Read the model definition and answer for the solid it produces. Units are mm, in the model's axes. Face numbers are marked on the shaded views. A direction names the side the tool comes from. Round coordinates to 2 decimals unless told otherwise and drop trailing zeros. Write each loop counter-clockwise with the first axis right and the second up, starting at its lowest first coordinate (ties: lowest second). Pieces come first, ordered by that corner, then holes.
from build123d import *

# Parameters (mm, degrees)
F0_W     = 75
F0_H     = 25
F0_R     = 1.75
F1_DEPTH = 2
F2_W     = 30
F2_H     = 25
F2_R     = 2.25
F3_DEPTH = 12
F4_DEPTH = 4
F5_R     = 5


with BuildPart() as f1:
    # F0 (on Top) → F1 (new body, symmetric)
    with BuildSketch(Plane.XY):
        Rectangle(F0_W, F0_H)
        with Locations((-30, 0)):
            Circle(F0_R, mode=Mode.SUBTRACT)
        with Locations((-20, 0)):
            Circle(F0_R, mode=Mode.SUBTRACT)
    extrude(amount=F1_DEPTH, both=True)

    # F2 (on face) → F3 (join)
    with BuildSketch(Plane(origin=(0, 0, -2), x_dir=(1, 0, 0), z_dir=(0, 0, -1))):
        with Locations((22.5, 0)):
            Rectangle(F2_W, F2_H)
        with Locations((15, 0)):
            Circle(F2_R, mode=Mode.SUBTRACT)
        with Locations((30, 0)):
            Circle(F2_R, mode=Mode.SUBTRACT)
    extrude(amount=F3_DEPTH)

    # F4 (cut, through all): faces of the model
    f4_faces = [f1.faces().sort_by_distance(p)[0] for p in [
        (15, 0, -2),
        (30, 0, -2),
    ]]
    extrude(f4_faces, amount=-F4_DEPTH, mode=Mode.SUBTRACT)

    # F5
    f5_edges = [f1.edges().sort_by_distance(p)[0] for p in [
        (-37.5, 12.5, 0),
        (-37.5, -12.5, 0),
        (7.5, 0, -2),
        (37.5, -12.5, -6),
        (37.5, 12.5, -6),
    ]]
    fillet(f5_edges, radius=F5_R)


solid = f1.part
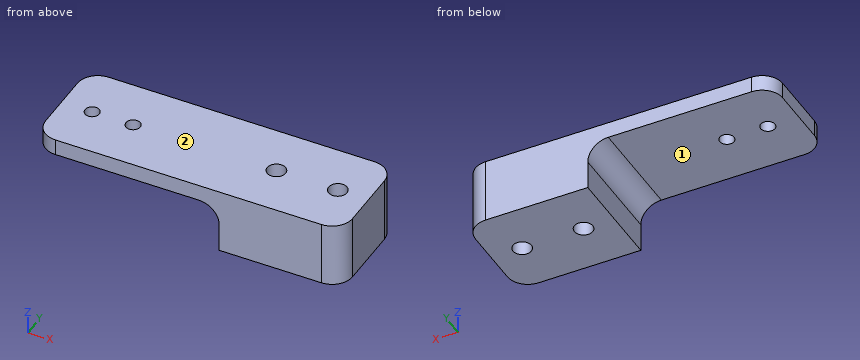
Q1. Section A-A (x = -30) is taken. Determine the outline of the cut face in (y, z).
Verdict:
outline: (-12.5, -2) - (-1.75, -2) - (-1.75, 2) - (-12.5, 2) - close; (1.75, -2) - (12.5, -2) - (12.5, 2) - (1.75, 2) - close
Q2. Section D-D (z = -12.5) is taken. Determine the outline of the cut face in (x, y).
Verdict:
outline: (7.5, -12.5) - (32.5, -12.5) arc R5 ccw to (37.5, -7.5) - (37.5, 7.5) arc R5 ccw to (32.5, 12.5) - (7.5, 12.5) - close; hole circle Ø4.5 at (15, 0); hole circle Ø4.5 at (30, 0)
Q3. Section C-C (z = -0.25) is taken. Determine the outline of the cut face in (x, y), then the cut area to 3 significant figures.
Verdict:
outline: (-37.5, -7.5) arc R5 ccw to (-32.5, -12.5) - (32.5, -12.5) arc R5 ccw to (37.5, -7.5) - (37.5, 7.5) arc R5 ccw to (32.5, 12.5) - (-32.5, 12.5) arc R5 ccw to (-37.5, 7.5) - close; hole circle Ø3.5 at (-30, 0); hole circle Ø3.5 at (-20, 0); hole circle Ø4.5 at (15, 0); hole circle Ø4.5 at (30, 0)
area: 1,800 mm2
Q4. Straight lines are drawn through the part: probe 1 along X at (y, z) = (0, -10.25); probe 2 along Y at (x, z) = (30, -8.75); probe 3 along X at (y, z) = (2, -11.5). For each, find the intervals that lie inside material, in ascending order.
Verdict:
probe 1: x = 7.5 to 12.75, 17.25 to 27.75, 32.25 to 37.5
probe 2: y = -12.5 to -2.25, 2.25 to 12.5
probe 3: x = 7.5 to 13.97, 16.03 to 28.97, 31.03 to 37.5
Q5. Which of the six approach directions +Z, -Z, +X, -X, +Y, -Y give full straight-line access (tool end or side, diameter ignored) to the marked faces 1 and 2?
Verdict:
face 1: -Z, -X, +Y, -Y
face 2: +Z, +X, -X, +Y, -Y
Q6. Flat-ended cylindrical pins translate along their axes: pin 1 Ø12.5 at (x, y) = (-12.5, -3) entering from -Z; pin 2 Ø5 at (y, z) = (-5.5, -9) entering from -X; pin 3 Ø4 at (x, y) = (30, 0) entering from +Z; pin 4 Ø7 at (x, y) = (15, 0) entering from -Z. Find the tip coordinate at first contact, or state that the pin passes through.
Verdict:
pin 1: stops at z = -2
pin 2: stops at x = 7.47
pin 3: passes through
pin 4: stops at z = -14
Q7. Section B-B (y = 0) is taken. Determine the outline of the cut face in (x, z), then the cut area to 3 significant figures.
Verdict:
outline: (-37.5, -2) - (-31.75, -2) - (-31.75, 2) - (-37.5, 2) - close; (-28.25, -2) - (-21.75, -2) - (-21.75, 2) - (-28.25, 2) - close; (-18.25, -2) - (2.5, -2) arc R5 cw to (7.5, -7) - (7.5, -14) - (12.75, -14) - (12.75, 2) - (-18.25, 2) - close; (17.25, -14) - (27.75, -14) - (27.75, 2) - (17.25, 2) - close; (32.25, -14) - (37.5, -14) - (37.5, 2) - (32.25, 2) - close
area: 493 mm2
